from build123d import *

# Parameters (mm, degrees)
F0_W     = 17
F0_H     = 4
F1_DEPTH = 2
F2_W     = 17
F2_H     = 2
F2_W_2   = 7
F3_DEPTH = 10
F4_R     = 0.2


with BuildPart() as f1:
    # F0 (on Top) → F1 (new body)
    with BuildSketch(Plane.XY):
        with Locations((-8.5, 2)):
            Rectangle(F0_W, F0_H)
    extrude(amount=F1_DEPTH)

    # F2 (on face) → F3 (join)
    with BuildSketch(Plane(origin=(0, 0, 0), x_dir=(1, 0, 0), z_dir=(0, 0, -1))):
        with Locations((-8.5, -5)):
            Rectangle(F2_W, F2_H)
        with Locations((-13.5, 1)):
            Rectangle(F2_W_2, F2_H)
    extrude(amount=-F3_DEPTH)

    # F4
    f4_edges = [f1.edges().sort_by_distance(p)[0] for p in [
        (-13.5, -2, 10),
        (-13.5, 0, 10),
        (-8.5, 4, 10),
        (-8.5, 6, 10),
    ]]
    fillet(f4_edges, radius=F4_R)


solid = f1.part
Geometry: final body of the model. Coordinates: model frame, mm. A direction names the side the tool comes from. Give positions to 0.01 mm unless a question says otherwise; leave off trailing zeros. Order: outer loops, then holes, each group sorted by start corner. A loop starts at its lowest first (then second) coordinate and runs counter-clockwise, first axis right, second up. Notation, with made-up numbers: (-19, -32.75) -> (8, -32.75) arc R28 ccw to (8, -6.75) -> close; hole circle Ø4 at (78.25, 55.5). An arc over 180 degrees is marked (long way). Write each question's results on one line, items separated by ' | '.
1) Draft query along Y for faces 1 (the face through (-14, 0, 6)), 2 (the face through (-9, 2, 2)), 3 (the face through (-10, -1, 5)), 4 (the face through (-5, 0, 1)). Return one class per face: released by +Y, released by -Y, zero draft, split by the parting line, or undercut.
Geometry says:
face 1: undercut | face 2: undercut | face 3: zero draft | face 4: released by -Y
2) Line query: line 1 along Y through (x, z) = (-12.5, 6); line 2 along Y through (x, z) = (-5.75, 4); line 3 along Z through (x, y) = (-4.75, 1.75). Output: solid intervals per line, ascending.
Geometry says:
line 1: y = -2 to 0, 4 to 6 | line 2: y = 4 to 6 | line 3: z = 0 to 2
3) Cut plane A-A (z = 8). Output: boundary loops of the cut face in (x, y).
Geometry says:
outline: (-17, -2) -> (-10, -2) -> (-10, 0) -> (-17, 0) -> close; (-17, 4) -> (0, 4) -> (0, 6) -> (-17, 6) -> close
4) First-contact query: pin 1 Ø0.6 at (y, z) = (-0.5, 4) entering from +X; pin 2 Ø1.6 at (x, z) = (-6.5, 1) entering from -Y; pin 3 Ø4 at (y, z) = (1.5, 2.5) entering from -X; pin 4 Ø1.2 at (x, y) = (-8.5, 1.5) entering from +Z. Flat tips, straight axial feed; report the tip coordinate or a pass-through.
Geometry says:
pin 1: stops at x = -10 | pin 2: stops at y = 0 | pin 3: stops at x = -17 | pin 4: stops at z = 2
5) Cut plane B-B (x = -9.75). Output: boundary loops of the cut face in (y, z), and give its area (3 significant figures).
Geometry says:
outline: (0, 0) -> (6, 0) -> (6, 9.8) arc R0.2 ccw to (5.8, 10) -> (4.2, 10) arc R0.2 ccw to (4, 9.8) -> (4, 2) -> (0, 2) -> close | area: 28.0 mm²
6) Cut plane D-D (y = -1). Output: boundary loops of the cut face in (x, z), and give its area (3 significant figures).
Geometry says:
outline: (-17, 0) -> (-10, 0) -> (-10, 10) -> (-17, 10) -> close | area: 70.0 mm²
7) Set-up query: faces 5 (the face through (-9, 5, 10)), 6 (the face through (-9, 4, 6)). Return all of +Z, -Z, +X, -X, +Y, -Y with unobstructed straight access to the full face (end or side cutting, diameter ignored); none if empty.
Geometry says:
face 5: +Z, +X, -X, +Y, -Y | face 6: +Z, +X, -X
8) Cut plane C-C (z = 1.25). Output: boundary loops of the cut face in (x, y), and give its area (3 significant figures).
Geometry says:
outline: (-17, -2) -> (-10, -2) -> (-10, 0) -> (0, 0) -> (0, 6) -> (-17, 6) -> close | area: 116 mm²
